from build123d import *

# Parameters (mm, degrees)
SKETCH1_R            = 114.3
BASE_DEPTH           = 5.334
SKETCH2_R            = 63.5
CENTER_CUT_DEPTH     = 162.732592745
SENSOR_CUTOUTS_DEPTH = 162.732592745
SKETCH7_W            = 30.48
SKETCH7_H            = 48.26
CUT_EXTRUDE2_DEPTH   = 162.891213524
HOLE3_OUTLINE_R      = 3.175
HOLE3_DEPTH          = 5.334


# Read off the part's stored shape, not the designer's step: Hole3
with BuildPart() as part:
    # Sketch1 → Base (new body)
    with BuildSketch(Plane(origin=(0, 0, 0), x_dir=(1, 0, 0), z_dir=(0, 1, 0))):
        with Locations(Location((0, 0, 0), (0, 0, 270))):
            Circle(SKETCH1_R)
    extrude(amount=BASE_DEPTH)

    # Sketch2 → Center Cut (cut, through all)
    with BuildSketch(Plane(origin=(0, 5.334, 0), x_dir=(1, 0, 0), z_dir=(0, 1, 0))):
        with Locations(Location((0, 0, 0), (0, 0, 270))):
            Circle(SKETCH2_R)
    extrude(amount=-CENTER_CUT_DEPTH, mode=Mode.SUBTRACT)

    # Sketch3 → Sensor Cutouts (cut, through all)
    with BuildSketch(Plane(origin=(0, 5.334, 0), x_dir=(1, 0, 0), z_dir=(0, 1, 0))):
        with BuildLine():
            Line((5.832770158, 114.151078805), (2.5, 95.25))
            Line((2.5, 95.25), (2.5, 86.614))
            Line((2.5, 86.614), (-2.5, 86.614))
            Line((-2.5, 86.614), (-2.5, 95.25))
            Line((-2.5, 95.25), (-5.832770158, 114.151078805))
            ThreePointArc((-5.832770158, 114.151078805), (0, 114.3), (5.832770158, 114.151078805))
        make_face()
        with BuildLine():
            Line((20.28, 95.25), (23.218811767, 111.916829745))
            ThreePointArc((23.218811767, 111.916829745), (17.647544886, 112.929421142), (12.032965395, 113.664848321))
            Line((12.032965395, 113.664848321), (15.28, 95.25))
            Line((15.28, 95.25), (15.28, 86.614))
            Line((15.28, 86.614), (20.28, 86.614))
            Line((20.28, 86.614), (20.28, 95.25))
        make_face()
        with BuildLine():
            Line((-20.28, 95.25), (-23.218811767, 111.916829745))
            ThreePointArc((-23.218811767, 111.916829745), (-17.647544886, 112.929421142), (-12.032965395, 113.664848321))
            Line((-12.032965395, 113.664848321), (-15.28, 95.25))
            Line((-15.28, 95.25), (-15.28, 86.614))
            Line((-15.28, 86.614), (-20.28, 86.614))
            Line((-20.28, 86.614), (-20.28, 95.25))
        make_face()
        Polygon((86.36, 45.56), (114.3, 50.486575841), (114.3, 35.633424159), (86.36, 40.56), (77.724, 40.56), (77.724, 45.56), align=None)
        Polygon((86.36, 61.99), (114.3, 66.916575841), (114.3, 52.063424159), (86.36, 56.99), (77.724, 56.99), (77.724, 61.99), align=None)
        Polygon((86.36, 29.13), (114.3, 34.056575841), (114.3, 19.203424159), (86.36, 24.13), (77.724, 24.13), (77.724, 29.13), align=None)
        with BuildLine():
            Line((15.28, -95.25), (15.28, -86.614))
            Line((15.28, -86.614), (20.28, -86.614))
            Line((20.28, -86.614), (20.28, -95.25))
            Line((20.28, -95.25), (23.218811767, -111.916829745))
            ThreePointArc((23.218811767, -111.916829745), (17.647544886, -112.929421142), (12.032965395, -113.664848321))
            Line((12.032965395, -113.664848321), (15.28, -95.25))
        make_face()
        with BuildLine():
            Line((2.5, -86.614), (2.5, -95.25))
            Line((2.5, -95.25), (5.832770158, -114.151078805))
            ThreePointArc((5.832770158, -114.151078805), (0, -114.3), (-5.832770158, -114.151078805))
            Line((-5.832770158, -114.151078805), (-2.5, -95.25))
            Line((-2.5, -95.25), (-2.5, -86.614))
            Line((-2.5, -86.614), (2.5, -86.614))
        make_face()
        with BuildLine():
            Line((-15.28, -86.614), (-15.28, -95.25))
            Line((-15.28, -95.25), (-12.032965395, -113.664848321))
            ThreePointArc((-12.032965395, -113.664848321), (-17.647544886, -112.929421142), (-23.218811767, -111.916829745))
            Line((-23.218811767, -111.916829745), (-20.28, -95.25))
            Line((-20.28, -95.25), (-20.28, -86.614))
            Line((-20.28, -86.614), (-15.28, -86.614))
        make_face()
        Polygon((-77.724, 24.13), (-86.36, 24.13), (-114.3, 19.203424159), (-114.3, 34.056575841), (-86.36, 29.13), (-77.724, 29.13), align=None)
        Polygon((-77.724, 40.56), (-86.36, 40.56), (-114.3, 35.633424159), (-114.3, 50.486575841), (-86.36, 45.56), (-77.724, 45.56), align=None)
        Polygon((-77.724, 56.99), (-86.36, 56.99), (-114.3, 52.063424159), (-114.3, 66.916575841), (-86.36, 61.99), (-77.724, 61.99), align=None)
    extrude(amount=-SENSOR_CUTOUTS_DEPTH, mode=Mode.SUBTRACT)

    # Sketch7 → Cut-Extrude2 (cut, through all)
    with BuildSketch(Plane.XZ.offset(5.334)):
        with Locations((-116.84, 0)):
            Rectangle(SKETCH7_W, SKETCH7_H)
        with Locations((116.84, 0)):
            Rectangle(SKETCH7_W, SKETCH7_H)
    extrude(amount=-CUT_EXTRUDE2_DEPTH, mode=Mode.SUBTRACT)

    # Hole3 outline → Hole3 (cut)
    with BuildSketch(Plane(origin=(0, 0, 0), x_dir=(1, 0, 0), z_dir=(0, 1, 0))):
        with Locations((-54.61, -78.74)):
            Circle(HOLE3_OUTLINE_R)
        with Locations((54.61, -78.74)):
            Circle(HOLE3_OUTLINE_R)
        with Locations((54.61, 78.74)):
            Circle(HOLE3_OUTLINE_R)
        with Locations((-54.61, 78.74)):
            Circle(HOLE3_OUTLINE_R)
    extrude(amount=HOLE3_DEPTH, mode=Mode.SUBTRACT)


solid = part.part
Can you work these out from the model? Positions are in its coordinate system, mm. A direction names the side the tool comes from. Give positions to 0.01 mm unless a question says otherwise; leave off trailing zeros. Loops run counter-clockwise (first coordinate to the right, second up) from the corner with the lowest first, then second, coordinate; pieces in that order, holes last. Notation, with made-up numbers: M 72.25,44 L 116.25,44 A20 ccw 116.25,58 Z; hole C -39.5,31 d7. An arc over 180 degrees is marked long. One line per item, written item: value.
1) Please list where these lines run through material, in increasing order: line 1 (X direction, y = 3.1, z = 0); line 2 (X direction, y = 1.95, z = 80.5); line 3 (Z direction, x = 91, y = 1.05).
Geometry check:
line 1: x = -101.6 to -63.5, 63.5 to 101.6
line 2: x = -81.14 to -57.25, -51.97 to 51.97, 57.25 to 81.14
line 3: z = -69.16 to -62.81, -56.17 to -46.38, -39.74 to -29.95, -23.31 to 69.16
2) Imagine slicing it at D-D on z = -78.74. Write out the boundary of the cut face in (x, y) (3 decimals).
Geometry check:
outline: M -82.852,0 L -57.785,0 L -57.785,5.334 L -82.852,5.334 Z; M -51.435,0 L 51.435,0 L 51.435,5.334 L -51.435,5.334 Z; M 57.785,0 L 82.852,0 L 82.852,5.334 L 57.785,5.334 Z
3) Thinking about a two-plate mould opening in X: for faces 1 (the face through (-77.724, 3, -60)), 2 (the face through (-82, 3, -29.13)), 3 (the face through (102.03, 2.63, -51.52)), 4 (the face through (-61.99, 2.7, -13.77)), which applies, +X half, -X half, draft (parallel to the pull), parting line (faces both ways), or undercut?
Geometry check:
face 1: -X half
face 2: draft
face 3: +X half
face 4: undercut
4) On a 3-axis mill with a long thin cutter (end or side, diameter ignored), from which of +Z, -Z, +X, -X, +Y, -Y can I reach the whole of each face in a straight line? I mean faces 5 (the face through (-90.754, 2.704, -62.765)), 6 (the face through (2.5, 3, 91)), 7 (the face through (18, 3, -86.614)). Say none if no direction works.
Geometry check:
face 5: -X, +Y, -Y
face 6: +Z, +Y, -Y
face 7: -Z, +Y, -Y
5) Imagine slicing it at A-A on z = 0. Write out the boundary of the cut face in (x, y), and give its area (3 significant figures).
Geometry check:
outline: M -101.6,0 L -63.5,0 L -63.5,5.33 L -101.6,5.33 Z; M 63.5,0 L 101.6,0 L 101.6,5.33 L 63.5,5.33 Z
area: 406 mm²
6) Imagine slicing it at B-B on x = 27. Write out the boundary of the cut face in (y, z).
Geometry check:
outline: M 0,-111.07 L 5.33,-111.07 L 5.33,-57.47 L 0,-57.47 Z; M 0,57.47 L 5.33,57.47 L 5.33,111.07 L 0,111.07 Z
7) Imagine slicing it at C-C on x = -54.61. Write out the boundary of the cut face in (y, z) (3 decimals).
Geometry check:
outline: M 0,-100.41 L 5.334,-100.41 L 5.334,-81.915 L 0,-81.915 Z; M 0,-75.565 L 5.334,-75.565 L 5.334,-32.404 L 0,-32.404 Z; M 0,32.404 L 5.334,32.404 L 5.334,75.565 L 0,75.565 Z; M 0,81.915 L 5.334,81.915 L 5.334,100.41 L 0,100.41 Z
8) I'm going to push flat-ended pins straight in: pin 1 (1.6 mm diameter, centred on x = -109, y = 2, fed in from -Z); pin 2 (2.5 mm diameter, centred on y = 3, z = 92.5, fed in from +X); pin 3 (2.5 mm diameter, centred on y = 3.5, z = -43.5, fed in from +X); pin 4 (5 mm diameter, centred on x = 54.61, z = 78.74, fed in from +Y). Where does each tip first touch, or does it pass through?
Geometry check:
pin 1: stops at z = -36.71
pin 2: stops at x = 68.83
pin 3: stops at x = 77.72
pin 4: passes through
